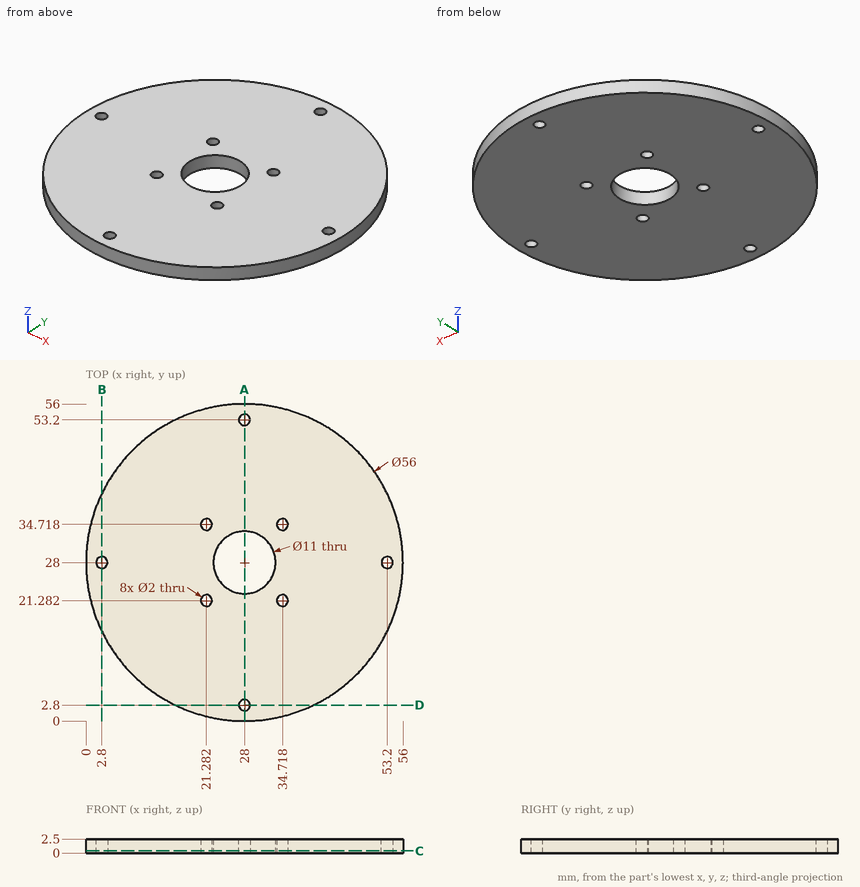
Input: dimensioned drawing with shaded views. Units: mm. Origin: part minimum x, y, z. Give positions to 0.01 mm unless a question says otherwise; leave off trailing zeros. Write each loop counter-clockwise with the first axis right and the second up, starting at its lowest first coordinate (ties: lowest second). Pieces come first, ordered by that corner, then holes. Notation, with made-up numbers: (64, -13) - (96, -13) arc R12 cw to (96, 2) - close; hole circle Ø2 at (82, 39.5). An arc over 180 degrees is marked (long way). One line per item, written item: value. Start each with the question number.
Q1. Section query A-A, the plane x = 28. Return the cut outline in (y, z).
Q2. Material intervals for probe 1 along Y at (x, z) = (28, 1.8); probe 2 along Y at (x, z) = (25.5, 0.9); probe 3 along X at (y, z) = (26.5, 0.5), sorted ascending. Write a range as from..to.
Q3. First-contact query: pin 1 Ø1.2 at (x, y) = (2.8, 28) entering from -Z; pin 2 Ø1.5 at (x, z) = (29, 1) entering from -Y. Flat tips, straight axial feed; report the tip coordinate or a pass-through.
Q4. Section query B-B, the plane x = 2.8. Return the cut outline in (y, z) (1 decimal).
Q5. Section query C-C, the plane z = 0.4. Count the separate pieces of the cut face and the enclosed holes in it, then the cut area to 3 significant figures.
Answer:
1. outline: (0, 0) - (1.8, 0) - (1.8, 2.5) - (0, 2.5) - close; (3.8, 0) - (22.5, 0) - (22.5, 2.5) - (3.8, 2.5) - close; (33.5, 0) - (52.2, 0) - (52.2, 2.5) - (33.5, 2.5) - close; (54.2, 0) - (56, 0) - (56, 2.5) - (54.2, 2.5) - close
2. probe 1: y = 0..1.8, 3.8..22.5, 33.5..52.2, 54.2..56
2. probe 2: y = 0.11..23.1, 32.9..55.89
2. probe 3: x = 0.04..22.71, 33.29..55.96
3. pin 1: passes through
3. pin 2: stops at y = 0
4. outline: (15.8, 0) - (27, 0) - (27, 2.5) - (15.8, 2.5) - close; (29, 0) - (40.2, 0) - (40.2, 2.5) - (29, 2.5) - close
5. separate pieces: 1
5. enclosed holes: 9
5. area: 2,340 mm2
